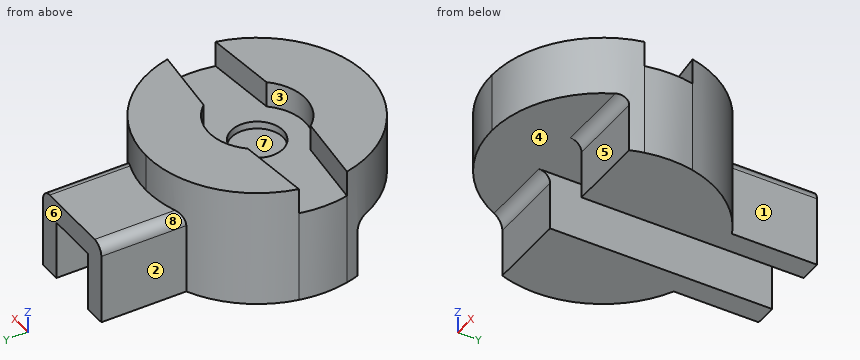
Autodesk Fusion 360 part; units mm, degrees
sketch "Sketch1" plane through (0, 0, 0) normal (0, 0, 1) x (1, 0, 0)
  circle A0 centre (0, 0) radius 6.5
  line L0 (-15, 0) -> (15, 0) construction
  line L1 (0, 15) -> (0, -15) construction
  arc A1 (-14.6437, -3.25) -> (0, -15) centre (0, 0) ccw
  arc A2 (14.6437, -3.25) -> (14.6437, 3.25) centre (0, 0) ccw
  arc A3 (-14.6437, 3.25) -> (-14.6437, -3.25) centre (0, 0) ccw
  arc A4 (0, 15) -> (-14.6437, 3.25) centre (0, 0) ccw
  arc A5 (0, -15) -> (14.6437, -3.25) centre (0, 0) ccw
  arc A6 (14.6437, 3.25) -> (0, 15) centre (0, 0) ccw
  line L2 (4.9181, 4.25) -> (4.9181, -4.25)
  line L3 (14.6437, 3.25) -> (14.6437, -3.25)
  line L4 (4.9181, -4.25) -> (14.6437, -3.25)
  line L5 (4.9181, 4.25) -> (14.6437, 3.25)
  line L6 (-14.6437, 3.25) -> (-14.6437, -3.25)
  line L7 (-4.9181, -4.25) -> (-14.6437, -3.25)
  line L8 (-4.9181, 4.25) -> (-4.9181, -4.25)
  line L9 (-4.9181, 4.25) -> (-14.6437, 3.25)
  circle A7 centre (0, 0) radius 3.5
  dimension "d1" = 30
  dimension "d2" = 13
  dimension "d5" = 6.5
  dimension "d6" = 8.5
  dimension "d25" = 7
extrude "Extrude1" add sketch "Sketch1" along normal blind 16 contours A0 L2 | A0 L3 L4 L5 | A0 L2 L8 | A0 A4 A6 L5 L9 | A0 A1 A5 L4 L7 | A0 L8 | A0 L6 L7 L9 | A2 L3 | A3 L6 | A7
extrude "Extrude2" cut sketch "Sketch1" against normal blind 3.5 from surface at 16 contours A0 L2 | A0 L3 L4 L5 | A0 L2 L8 | A0 L8 | A0 L6 L7 L9 | A2 L3 | A3 L6 | A7
sketch "Sketch2" plane through (0, 0, 0) normal (0, 0, 1) x (1, 0, 0)
  arc A0 (-14.6437, -3.25) -> (0, -15) centre (0, 0) ccw
  arc A1 (0, -15) -> (14.6437, -3.25) centre (0, 0) ccw
  arc A2 (14.6437, -3.25) -> (14.6437, 3.25) centre (0, 0) ccw
  arc A3 (14.6437, 3.25) -> (0, 15) centre (0, 0) ccw
  arc A4 (0, 15) -> (-14.6437, 3.25) centre (0, 0) ccw
  arc A5 (-14.6437, 3.25) -> (-14.6437, -3.25) centre (0, 0) ccw
  line L0 (3.5, 15) -> (-3.5, 15)
  line L1 (-3.5, 15) -> (-3.5, -15)
  line L2 (-3.5, -15) -> (3.5, -15)
  line L3 (3.5, -15) -> (3.5, 15)
  line L4 (3.5, 15) -> (-3.5, -15) construction
  line L5 (-3.5, 15) -> (3.5, -15) construction
  dimension "d29" = 7
  dimension "d30" = 30
extrude "Extrude5" cut sketch "Sketch1" against normal blind 1 from surface at 12.5 contours A7
extrude "Extrude6" cut sketch "Sketch2" along normal blind 8 contours A0 A1 A3 A4 L1 L3
sketch "Sketch3" plane through (0, 0, 0) normal (0, 0, 1) x (1, 0, 0)
  arc A0 (0, 15) -> (-14.6437, 3.25) centre (0, 0) ccw construction
  arc A1 (-14.6437, 3.25) -> (-14.6437, -3.25) centre (0, 0) ccw construction
  arc A2 (-14.6437, -3.25) -> (0, -15) centre (0, 0) ccw construction
  arc A3 (0, -15) -> (14.6437, -3.25) centre (0, 0) ccw construction
  arc A4 (14.6437, 3.25) -> (0, 15) centre (0, 0) ccw construction
  arc A5 (14.6437, -3.25) -> (14.6437, 3.25) centre (0, 0) ccw construction
  line L0 (15, -15) -> (15, -5)
  line L1 (15, -5) -> (-15, -5)
  line L2 (-15, -5) -> (-15, -15)
  line L3 (0, 15) -> (0, 10) construction
  line L4 (6.5, 10) -> (6.5, 25)
  line L5 (6.5, 25) -> (-6.5, 25)
  line L6 (-6.5, 25) -> (-6.5, 10)
  line L7 (-11.1803, 10) -> (-6.5, 10) construction
  line L8 (6.5, 10) -> (11.1803, 10) construction
  line L9 (-6.5, 10) -> (0, 10)
  line L10 (0, 10) -> (6.5, 10)
  line L11 (3.5, 15) -> (-3.5, 15) construction
  line L12 (3.5, -15) -> (3.5, 15)
  line L13 (-3.5, -15) -> (3.5, -15) construction
  line L14 (-3.5, 15) -> (-3.5, -15)
  line L15 (15, -15) -> (-15, -15)
  line L16 (-3.5, 15) -> (-3.5, 25)
  line L17 (3.5, 15) -> (3.5, 25)
  dimension "d38" = 10
  dimension "d39" = 30
  dimension "d40" = 5
  dimension "d41" = 15
  dimension "d42" = 13
  dimension "d43" = 6.5
  dimension "d46" = 15
extrude "Extrude7 (1)" add sketch "Sketch3" along normal blind 11 contours L4 L5 L10 L12 L17 | L5 L9 L10 L12 L14 L16 L17 | L5 L6 L9 L14 L16
extrude "Extrude8" cut sketch "Sketch3" along normal blind 8 contours L0 L1 L12 L15 | L1 L12 L14 L15 | L1 L2 L14 L15 | L5 L9 L10 L12 L14 L16 L17
fillet "Fillet1" radius 1.5 2 edges at (6.5, 19.2593, 11) (-6.5, 19.2593, 11)
fillet "Fillet2" radius 1.5 2 edges at (8.8211, -5, 8) (-8.8211, -5, 8)
Geometry check sheet. Reference: the model listing, model coordinates, mm. Face numbers are marked on the shaded views. A direction names the side the tool comes from. Round coordinates to 2 decimals unless told otherwise and drop trailing zeros. Write each loop counter-clockwise with the first axis right and the second up, starting at its lowest first coordinate (ties: lowest second). Pieces come first, ordered by that corner, then holes. Notation, with made-up numbers: (-27, -18) -> (-12, -18) arc R34 ccw to (-12, 19) -> close; hole circle Ø9 at (62, -25.5). An arc over 180 degrees is marked (long way). Put each result on its own line as item: value.
1) Depth check by flat-ended pin: P1, Ø12, axis at x = 4.5, y = -3, coming from the +Z side; P2, Ø2, axis at y = 12, z = 2.5, coming from the -X side; P3, Ø4, axis at x = 5.5, z = 5.5, coming from the -Y side; P4, Ø3, axis at x = -10.5, z = 3, coming from the -Y side. Enter the tip coordinate at first touch or a pass-through.
Recorded:
P1: stops at z = 16
P2: stops at x = -10.2
P3: stops at y = -5.38
P4: stops at y = -5
2) Thickness scan on probe 1 along Y at (x, z) = (0, 11.9); probe 2 along X at (y, z) = (20.5, 7.75); probe 3 along Z at (x, y) = (4, -4.5). Record the ranges inside material, lowest first. Write a range as from..to.
Recorded:
probe 1: y = -15..-3.5, 3.5..15
probe 2: x = -6.5..-3.5, 3.5..6.5
probe 3: z = 0..12.5
3) Access from +Z, -Z, +X, -X, +Y, -Y to the whole of each face (thin tool, end or side, straight path). Record for the marked faces 4, 5, 6, 7 and 8.
Recorded:
face 4: -Z, -Y
face 5: -Z, +X, -X, -Y
face 6: +Z, -Z, +X, -X, +Y
face 7: +Z
face 8: +Z, -X, +Y
4) Cross-section at C-C, the plane x = 10. Enter the section's corners in (y, z), plus the area to 3 significant figures.
Recorded:
outline: (-11.18, 8) -> (-6.5, 8) arc R1.5 cw to (-5, 6.5) -> (-5, 0) -> (11.18, 0) -> (11.18, 16) -> (3.73, 16) -> (3.73, 12.5) -> (-3.73, 12.5) -> (-3.73, 16) -> (-11.18, 16) -> close
area: 283 mm2
5) Release check for a two-part mould opening along X. For the marked faces 1, 2 and 3 record: pulls with the +X half, pulls with the -X half, needs draft (parallel to the pull), parting line crosses it, or undercut.
Recorded:
face 1: pulls with the +X half
face 2: pulls with the -X half
face 3: undercut
6) Cross-section at A-A, the plane z = 4. Enter the section's corners in (x, y), plus the area to 3 significant figures.
Recorded:
outline: (-14.64, -3.25) arc R15 ccw to (-14.14, -5) -> (-3.5, -5) -> (-3.5, 25) -> (-6.5, 25) -> (-6.5, 13.52) arc R15 ccw to (-14.64, 3.25) arc R15 ccw to start; (3.5, -5) -> (14.14, -5) arc R15 ccw to (14.64, -3.25) arc R15 ccw to (14.64, 3.25) arc R15 ccw to (6.5, 13.52) -> (6.5, 25) -> (3.5, 25) -> close
area: 427 mm2
7) Cross-section at B-B, the plane y = 0. Enter the section's corners in (x, z), plus the area to 3 significant figures.
Recorded:
outline: (-15, 0) -> (-3.5, 0) -> (-3.5, 8) -> (3.5, 8) -> (3.5, 0) -> (15, 0) -> (15, 12.5) -> (3.5, 12.5) -> (3.5, 11.5) -> (-3.5, 11.5) -> (-3.5, 12.5) -> (-15, 12.5) -> close
area: 312 mm2
8) Cross-section at D-D, the plane z = 14. Enter the section's corners in (x, y), plus the area to 3 significant figures.
Recorded:
outline: (-14.64, -3.25) arc R15 ccw to (0, -15) arc R15 ccw to (14.64, -3.25) -> (4.92, -4.25) arc R6.5 cw to (-4.92, -4.25) -> close; (-14.64, 3.25) -> (-4.92, 4.25) arc R6.5 cw to (4.92, 4.25) -> (14.64, 3.25) arc R15 ccw to (0, 15) arc R15 ccw to start
area: 444 mm2
